from build123d import *

# Parameters (mm, degrees)
F0_W           = 48
F0_H           = 48
F1_DEPTH       = 48
F2_R           = 1
F3_R           = 1
F4_T1_DEPTH    = 46
F4_T3_DEPTH    = 46
F4_T5_DEPTH    = 46
F4_S9_W        = 1
F4_S9_H        = 1
F4_T10_DEPTH   = 1
F4_S15_W       = 1
F4_S15_H       = 1
F4_T16_DEPTH   = 1
F4_S21_W       = 1
F4_S21_H       = 1
F4_T22_DEPTH   = 1
F4_S27_W       = 1
F4_S27_H       = 1
F4_T28_DEPTH   = 1
F4_T32_ANGLE   = 90
F4_T34_ANGLE   = 90
F6_D           = 18
F6_CSINK_D     = 36
F6_CSINK_ANGLE = 90
F8_D           = 18
F8_CSINK_D     = 36
F8_CSINK_ANGLE = 90


# Not quite as in the source:
# - a fillet or chamfer that OpenCascade refuses, or shapes differently, is made with other operations: its cross-section is extruded or revolved along the edge and cut away or added


with BuildPart() as f1:
    # F0 (on Front) → F1 (new body)
    with BuildSketch(Plane.XZ):
        Rectangle(F0_W, F0_H)
    extrude(amount=F1_DEPTH)

    # F2
    f2_edges = [f1.edges().sort_by_distance(p)[0] for p in [
        (24, -24, 24),
    ]]
    fillet(f2_edges, radius=F2_R)

    # F3
    f3_edges = [f1.edges().sort_by_distance(p)[0] for p in [
        (-24, -24, 24),
        (-0.5, 0, 24),
        (-0.5, -48, 24),
    ]]
    fillet(f3_edges, radius=F3_R)

    # F4: fillet of radius 1 on 8 edges, made by hand

    # F4_s2 → F4_t1 (cut)
    with BuildSketch(Plane.XY.offset(-23)):
        with BuildLine():
            ThreePointArc((-23, -48), (-23.7071067812, -47.7071067812), (-24, -47))
            Line((-24, -47), (-24, -48))
            Line((-24, -48), (-23, -48))
        make_face()
        with BuildLine():
            ThreePointArc((-23, 0), (-23.7071067812, -0.2928932188), (-24, -1))
            Line((-24, -1), (-24, 0))
            Line((-24, 0), (-23, 0))
        make_face()
    extrude(amount=F4_T1_DEPTH, mode=Mode.SUBTRACT)

    # F4_s4 → F4_t3 (cut)
    with BuildSketch(Plane.YZ.offset(-23)):
        with BuildLine():
            ThreePointArc((0, -23), (-0.2928932188, -23.7071067812), (-1, -24))
            Line((-1, -24), (0, -24))
            Line((0, -24), (0, -23))
        make_face()
        with BuildLine():
            ThreePointArc((-48, -23), (-47.7071067812, -23.7071067812), (-47, -24))
            Line((-47, -24), (-48, -24))
            Line((-48, -24), (-48, -23))
        make_face()
    extrude(amount=F4_T3_DEPTH, mode=Mode.SUBTRACT)

    # F4_s6 → F4_t5 (cut)
    with BuildSketch(Plane.XZ.offset(1)):
        with BuildLine():
            ThreePointArc((-24, -23), (-23.7071067812, -23.7071067812), (-23, -24))
            Line((-23, -24), (-24, -24))
            Line((-24, -24), (-24, -23))
        make_face()
        with BuildLine():
            ThreePointArc((24, -23), (23.7071067812, -23.7071067812), (23, -24))
            Line((23, -24), (24, -24))
            Line((24, -24), (24, -23))
        make_face()
    extrude(amount=F4_T5_DEPTH, mode=Mode.SUBTRACT)


with BuildPart() as f4_tool8:
    # F4_s9 → F4_t10 (new body)
    with BuildSketch(Plane.XZ.offset(1)):
        with Locations((-23.5, 23.5)):
            Rectangle(F4_S9_W, F4_S9_H)
    extrude(amount=-F4_T10_DEPTH)

    # F4_s11 → F4_t12 (revolve, cut)
    with BuildSketch(Plane(origin=(-23, -1, 23), x_dir=(0.7071067812, 0, -0.7071067812), z_dir=(0.7071067812, 0, 0.7071067812))):
        with BuildLine():
            ThreePointArc((0, -1), (1, 0), (0, 1))
            Line((0, 1), (0, -1))
        make_face()
    revolve(axis=Axis((-23, -1, 23), (0, 1, 0)), mode=Mode.SUBTRACT)


with BuildPart() as f1_1:
    add(f1.part)

    # F4_t7: cut F4_tool8
    add(f4_tool8.part, mode=Mode.SUBTRACT)


with BuildPart() as f4_tool14:
    # F4_s15 → F4_t16 (new body)
    with BuildSketch(Plane.XZ.offset(47)):
        with Locations((-23.5, 23.5)):
            Rectangle(F4_S15_W, F4_S15_H)
    extrude(amount=F4_T16_DEPTH)

    # F4_s17 → F4_t18 (revolve, cut)
    with BuildSketch(Plane(origin=(-23, -47, 23), x_dir=(0.7071067812, 0, -0.7071067812), z_dir=(-0.7071067812, 0, -0.7071067812))):
        with BuildLine():
            ThreePointArc((0, -1), (1, 0), (0, 1))
            Line((0, 1), (0, -1))
        make_face()
    revolve(axis=Axis((-23, -47, 23), (0, -1, 0)), mode=Mode.SUBTRACT)


with BuildPart() as f1_2:
    add(f1_1.part)

    # F4_t13: cut F4_tool14
    add(f4_tool14.part, mode=Mode.SUBTRACT)


with BuildPart() as f4_tool20:
    # F4_s21 → F4_t22 (new body)
    with BuildSketch(Plane.XZ.offset(47)):
        with Locations((-23.5, -23.5)):
            Rectangle(F4_S21_W, F4_S21_H)
    extrude(amount=F4_T22_DEPTH)

    # F4_s23 → F4_t24 (revolve, cut)
    with BuildSketch(Plane(origin=(-23, -47, -23), x_dir=(0.7071067812, 0, 0.7071067812), z_dir=(0.7071067812, 0, -0.7071067812))):
        with BuildLine():
            ThreePointArc((0, -1), (1, 0), (0, 1))
            Line((0, 1), (0, -1))
        make_face()
    revolve(axis=Axis((-23, -47, -23), (0, -1, 0)), mode=Mode.SUBTRACT)


with BuildPart() as f1_3:
    add(f1_2.part)

    # F4_t19: cut F4_tool20
    add(f4_tool20.part, mode=Mode.SUBTRACT)


with BuildPart() as f4_tool26:
    # F4_s27 → F4_t28 (new body)
    with BuildSketch(Plane.XZ.offset(1)):
        with Locations((-23.5, -23.5)):
            Rectangle(F4_S27_W, F4_S27_H)
    extrude(amount=-F4_T28_DEPTH)

    # F4_s29 → F4_t30 (revolve, cut)
    with BuildSketch(Plane(origin=(-23, -1, -23), x_dir=(0.7071067812, 0, 0.7071067812), z_dir=(-0.7071067812, 0, 0.7071067812))):
        with BuildLine():
            ThreePointArc((0, -1), (1, 0), (0, 1))
            Line((0, 1), (0, -1))
        make_face()
    revolve(axis=Axis((-23, -1, -23), (0, 1, 0)), mode=Mode.SUBTRACT)


with BuildPart() as f1_4:
    add(f1_3.part)

    # F4_t25: cut F4_tool26
    add(f4_tool26.part, mode=Mode.SUBTRACT)

    # F4_s31 → F4_t32 (revolve, cut)
    with BuildSketch(Plane.XZ.offset(1)):
        with BuildLine():
            ThreePointArc((24, -23), (23.7071067812, -23.7071067812), (23, -24))
            Line((23, -24), (24, -24))
            Line((24, -24), (24, -23))
        make_face()
    revolve(axis=Axis((23, -1, -24), (0, 0, 1)), revolution_arc=F4_T32_ANGLE, mode=Mode.SUBTRACT)

    # F4_s33 → F4_t34 (revolve, cut)
    with BuildSketch(Plane.XZ.offset(47)):
        with BuildLine():
            ThreePointArc((24, -23), (23.7071067812, -23.7071067812), (23, -24))
            Line((23, -24), (24, -24))
            Line((24, -24), (24, -23))
        make_face()
    revolve(axis=Axis((23, -47, -24), (0, 0, -1)), revolution_arc=F4_T34_ANGLE, mode=Mode.SUBTRACT)

    # F6 (through all)
    with Locations(Plane.XY.offset(24)):
        with Locations((0, -24)):
            CounterSinkHole(F6_D / 2, F6_CSINK_D / 2, counter_sink_angle=F6_CSINK_ANGLE)

    # F8 (through all)
    with Locations(Plane(origin=(-24, 0, 0), x_dir=(0, -1, 0), z_dir=(-1, 0, 0))):
        with Locations((24, 0)):
            CounterSinkHole(F8_D / 2, F8_CSINK_D / 2, counter_sink_angle=F8_CSINK_ANGLE)


solid = f1_4.part
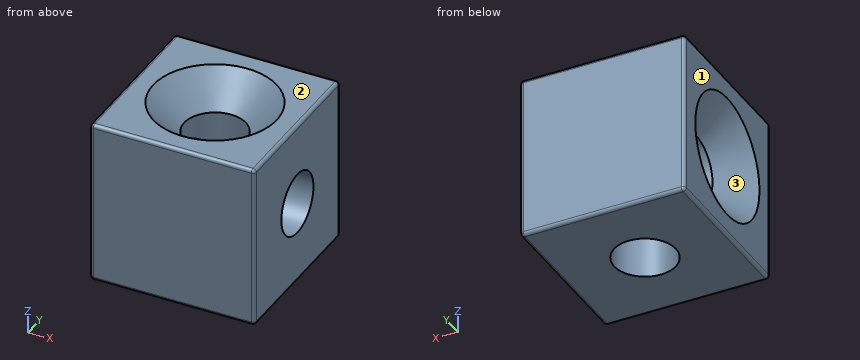
Can you work these out from the model? Positions are in its coordinate system, mm. Face numbers are marked on the shaded views. Give positions to 0.01 mm unless a question says otherwise; leave off trailing zeros. Loops run counter-clockwise (first coordinate to the right, second up) from the corner with the lowest first, then second, coordinate; pieces in that order, holes last. Notation, with made-up numbers: (63, -8) - (88, -8) arc R11 ccw to (88, 7) - close; hole circle Ø5 at (-2, -13). An arc over 180 degrees is marked (long way). One line per item, written item: value.
(1) If we section it at B-B, the plane z = 21: List the corners of the cut face in (x, y) for me, plus the area to 3 significant figures.
Verdict:
outline: (-24, -47) arc R1 ccw to (-23, -48) - (23, -48) arc R1 ccw to (24, -47) - (24, -1) arc R1 ccw to (23, 0) - (-23, 0) arc R1 ccw to (-24, -1) - close; hole circle Ø30 at (0, -24)
area: 1,600 mm^2
(2) If we section it at A-A, the plane y = -24: List the corners of the cut face in (x, z) for me.
Verdict:
outline: (-24, -23) arc R1 ccw to (-23, -24) - (-9, -24) - (-9, -9) - (-15, -9) - (-24, -18) - close; (-24, 18) - (-15, 9) - (-9, 9) - (-9, 15) - (-18, 24) - (-23, 24) arc R1 ccw to (-24, 23) - close; (9, -24) - (23, -24) arc R1 ccw to (24, -23) - (24, -9) - (9, -9) - close; (9, 9) - (24, 9) - (24, 23) arc R1 ccw to (23, 24) - (18, 24) - (9, 15) - close
(3) If we mould it in two halves opening along Z, with no side actions, what happens to the marked faces 1, 2 and 3? For each: released by +Z, released by -Z, zero draft, split by the parting line, or undercut.
Verdict:
face 1: zero draft
face 2: released by +Z
face 3: undercut
(4) I'm going to push flat-ended pins straight in: pin 1 (1.5 mm diameter, centred on x = 12.5, y = -21, fed in from +Z); pin 2 (3 mm diameter, centred on y = -9.5, z = 7.5, fed in from -X); pin 3 (20.5 mm diameter, centred on y = -24, z = 0, fed in from -X). Where does each tip first touch, or does it pass through?
Verdict:
pin 1: z = 19.6
pin 2: x = -23.82
pin 3: x = -16.25
(5) I need wall thicknesses on line 1 along Y through (x, z) = (0, 7); line 2 along Z through (x, y) = (19, -24); line 3 along X through (y, z) = (-41, -0.5). Which ranges of each line are inside material? Lowest first, please.
Verdict:
line 1: -48 to -33, -15 to 0
line 2: -24 to -9, 9 to 24
line 3: -23.01 to 24
